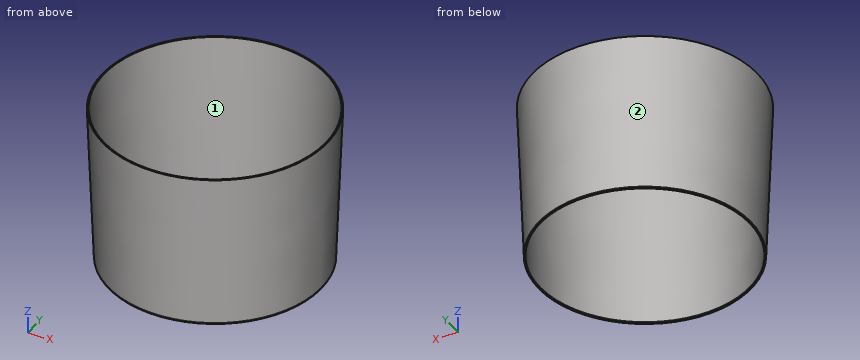
Autodesk Inventor part; units mm, degrees
ref_plane "YZ Plane" through (0, 0, 0) normal (1, 0, 0) x (0, 1, 0)
ref_plane "XZ Plane" through (0, 0, 0) normal (0, 1, 0) x (-1, 0, 0)
ref_plane "XY Plane" through (0, 0, 0) normal (0, 0, 1) x (1, 0, 0)
sketch "Skizze3" plane through (0, 0, 0) normal (0, 0, 1) x (1, 0, 0)
  line L0 (-201.6, 0) -> (201.6, 0)
  line L1 (0, -201.6) -> (0, 201.6)
  circle A0 centre (0, 0) radius 144
  dimension "d4" = 288
extrude "Extrusion2" add sketch "Skizze3" along normal blind 210 draft 2.25
sketch "Skizze4" plane through (0, 0, 210) normal (0, 0, 1) x (1, 0, 0)
  circle A0 centre (0, 0) radius 150.2509
  circle A1 centre (0, 0) radius 152.2509
  dimension "d7" = 2
extrude "Extrusion3" cut sketch "Skizze4" against normal blind 210 draft -2.25 contours A0
sketch "Skizze5" plane through (0, 0, 0) normal (0, 0, -1) x (-1, 0, 0)
  circle A0 centre (0, 0) radius 144
  circle A1 centre (0, 0) radius 144
  circle A2 centre (0, 0) radius 142
extrude "Extrusion4" add sketch "Skizze5" along normal blind 2
properties part number "Abdeckungsrohr"
Geometry: final body of the model. Coordinates: model frame, mm. Face numbers are marked on the shaded views. Give positions to 0.01 mm unless a question says otherwise; leave off trailing zeros. Loops run counter-clockwise (first coordinate to the right, second up) from the corner with the lowest first, then second, coordinate; pieces in that order, holes last. Notation, with made-up numbers: (1.5, 35.5) - (32.5, 35.5) arc R30 cw to (32.5, 68.5) - close; hole circle Ø5 at (-32.5, 44). An arc over 180 degrees is marked (long way). One line per question, with ' | ' between items. Start each with the question number.
(1) Contact query for flat-ended pins moving along their axis: pin 1 (1 mm diameter, centred on y = 109.5, z = 35, fed in from +X); pin 2 (10 mm diameter, centred on x = -46, z = 163.5, fed in from -Y); pin 3 (4 mm diameter, centred on y = -75.5, z = 77, fed in from -X). Output: stop coordinate, or through.
(2) Section query B-B on z = 119.5. Return loops of the section in (x, y).
(3) Pull-direction query (X, two-part tool) for the marked faces 1 and 2; classes: released by +X, released by -X, zero draft, split by the parting line, or undercut.
(4) Ray query, line 1 (Y direction, x = 0, z = -0.95); line 2 (X direction, y = -39, z = 85.5). Return the intervals inside material, ascending. Write a range as from..to.
(5) Section query A-A on x = 0. Return loops of the section in (y, z), then the cut area to 3 significant figures.
The answers:
1) pin 1: x = 96.19 | pin 2: y = -144.74 | pin 3: x = -127.34
2) outline: circle Ø297.39 at (0, 0); hole circle Ø293.39 at (0, 0)
3) face 1: undercut | face 2: split by the parting line
4) line 1: -144..-142, 142..144 | line 2: -142.1..-140.03, 140.03..142.1
5) outline: (-152.25, 210) - (-144, 0) - (-144, -2) - (-142, -2) - (-142, 0) - (-150.25, 210) - close; (142, -2) - (144, -2) - (144, 0) - (152.25, 210) - (150.25, 210) - (142, 0) - close | area: 848 mm2
